Part model, mm, in its own coordinate system. Face numbers are marked on the shaded views. A direction names the side the tool comes from. Coordinates: 2 decimals unless noted, no trailing zeros. Loops run counter-clockwise (first coordinate to the right, second up) from the corner with the lowest first, then second, coordinate; pieces in that order, holes last. Notation, with made-up numbers: (81.5, 45) -> (99.5, 45) arc R20 ccw to (99.5, 76) -> close; hole circle Ø4 at (64, 14.25). An arc over 180 degrees is marked (long way). One line per question, with ' | ' between items. Start each with the question number.
1) 3-axis set-ups, long thin cutter, end or side, ignore diameter. For the marked faces 1, 2 and 3: which of +Z, -Z, +X, -X, +Y, -Y reach the whole face in a straight line?
2) Drop flat-ended pins along their axis: pin 1 (4 mm diameter, centred on y = -2, z = 8.5, fed in from -X); pin 2 (3 mm diameter, centred on x = -71.5, y = -6.5, fed in from -Z); pin 3 (5 mm diameter, centred on x = -70, y = 6, fed in from -Z); pin 4 (10 mm diameter, centred on x = -49.5, y = 3.5, fed in from +Z). Give the stop position or say it passes through.
3) Probe L1, parallel to Z at x = -36.5, y = -4.25; L2, parallel to Y at x = -24, z = 1.25; L3, parallel to Y at x = -92.5, z = 2.5. List the from-to ranges inside material, lowest first. Write a range as from..to.
4) Cut at A-A (x = -45). List the corners of the cut face in (y, z), plus the area to 3 significant figures.
from build123d import *

# Parameters (mm, degrees)
F2_SIZE = 3
F3_R    = 6


with BuildPart() as f1:
    # F0 (on Top) → F1 (revolve)
    with BuildSketch(Plane.XY):
        Polygon((-106, 0), (0, 0), (0, 9.5), (-33, 9.5), (-36, 11), (-84, 11), (-87, 8.5), (-106, 8.5), align=None)
    revolve(axis=Axis((-53, 0, 0), (1, 0, 0)))

    # F2
    f2_edges = [f1.edges().sort_by_distance(p)[0] for p in [
        (-106, -8.5, 0),
    ]]
    chamfer(f2_edges, length=F2_SIZE)

    # F3
    f3_edges = [f1.edges().sort_by_distance(p)[0] for p in [
        (-87, -8.5, 0),
        (-33, -9.5, 0),
    ]]
    fillet(f3_edges, radius=F3_R)


solid = f1.part
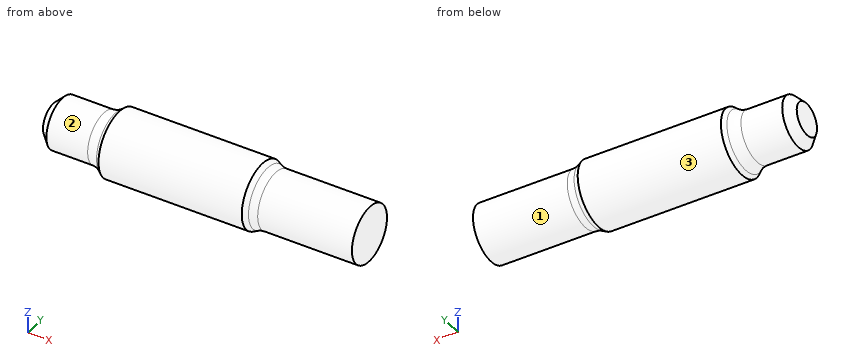
Reported:
1) face 1: +X | face 2: -X | face 3: +X, -X
2) pin 1: stops at x = -104.77 | pin 2: stops at z = -9.8 | pin 3: stops at z = -10.43 | pin 4: stops at z = 11
3) L1: z = -10.15..10.15 | L2: y = -9.42..9.42 | L3: y = -8.12..8.12
4) outline: circle Ø22 at (0, 0) | area: 380 mm²
